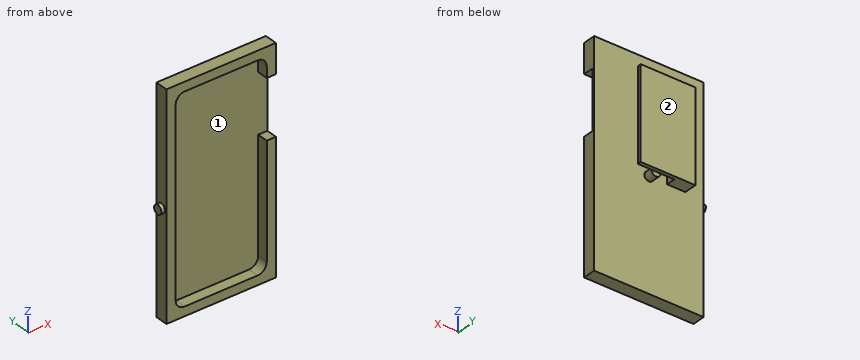
from build123d import *

# Parameters (mm, degrees)
F0_W      = 76.2
F0_H      = 152.4
F1_DEPTH  = 8.89
F3_DEPTH  = 7.62
F4_W      = 6.35
F4_H      = 40.64
F5_DEPTH  = 7.62
F7_DEPTH  = 2.54
F7_FACE_R = 3.175
F8_DEPTH  = 5.08
F9_R      = 3.175
F10_DEPTH = 6.35
F11_W     = 12.7
F11_H     = 63.5
F12_DEPTH = 8.89
F13_W     = 2.54
F13_H     = 63.5
F14_DEPTH = 25.4


with BuildPart() as f1:
    # F0 (on Front) → F1 (new body)
    with BuildSketch(Plane.XZ):
        with Locations((-38.1, 82.721622)):
            Rectangle(F0_W, F0_H)
    extrude(amount=F1_DEPTH)

    # F2 (on face) → F3 (cut)
    with BuildSketch(Plane.XZ.offset(8.89)):
        with BuildLine():
            ThreePointArc((-69.85, 19.221622), (-67.990128, 14.731494), (-63.5, 12.871622))
            Line((-63.5, 12.871622), (-12.7, 12.871622))
            ThreePointArc((-12.7, 12.871622), (-8.209872, 14.731494), (-6.35, 19.221622))
            Line((-6.35, 19.221622), (-6.35, 146.221622))
            ThreePointArc((-6.35, 146.221622), (-8.209872, 150.71175), (-12.7, 152.571622))
            Line((-12.7, 152.571622), (-50.255585, 152.571622))
            Line((-50.255585, 152.571622), (-63.5, 152.571622))
            ThreePointArc((-63.5, 152.571622), (-67.990128, 150.71175), (-69.85, 146.221622))
            Line((-69.85, 146.221622), (-69.85, 115.075722))
            Line((-69.85, 115.075722), (-69.85, 19.221622))
        make_face()
    extrude(amount=-F3_DEPTH, mode=Mode.SUBTRACT)

    # F4 (on face) → F5 (cut)
    with BuildSketch(Plane.XZ.offset(8.89)):
        with Locations((-3.175, 118.281622)):
            Rectangle(F4_W, F4_H)
    extrude(amount=-F5_DEPTH, mode=Mode.SUBTRACT)

    # F6 (on face) → F7 (cut)
    with BuildSketch(Plane(origin=(-76.2, 0, 0), x_dir=(0, -1, 0), z_dir=(-1, 0, 0))):
        with BuildLine():
            ThreePointArc((4.445, 76.371622), (6.64402, 77.326013), (7.548988, 79.545828))
            ThreePointArc((7.548988, 79.545828), (2.103956, 81.765643), (4.445, 76.371622))
        make_face()
    extrude(amount=-F7_DEPTH, mode=Mode.SUBTRACT)

    # F7_face (on face) → F8 (join)
    with BuildSketch(Plane(origin=(-73.66, -4.373988, 79.545828), x_dir=(0, -1, 0), z_dir=(-1, 0, 0))):
        Circle(F7_FACE_R)
    extrude(amount=F8_DEPTH)

    # F9 (on face) → F10 (join)
    with BuildSketch(Plane(origin=(0, 0, 0), x_dir=(-1, 0, 0), z_dir=(0, 1, 0))):
        with Locations((38.1, 82.721622)):
            Circle(F9_R)
    extrude(amount=F10_DEPTH)

    # F11 (on face) → F12 (join)
    with BuildSketch(Plane(origin=(0, 0, 0), x_dir=(-1, 0, 0), z_dir=(0, 1, 0))):
        with Locations((57.15, 114.471622)):
            Rectangle(F11_W, F11_H)
    extrude(amount=F12_DEPTH)

    # F13 (on face) → F14 (join)
    with BuildSketch(Plane.YZ.offset(-50.8)):
        with Locations((7.62, 114.471622)):
            Rectangle(F13_W, F13_H)
    extrude(amount=F14_DEPTH)


solid = f1.part
Here's how the part is built. I have some questions about the finished solid (model axes, mm). Face numbers are marked on the shaded views. Give positions to 0.01 mm unless a question says otherwise; leave off trailing zeros. Loops run counter-clockwise (first coordinate to the right, second up) from the corner with the lowest first, then second, coordinate; pieces in that order, holes last. Notation, with made-up numbers: (32.5, 73) -> (83.5, 73) arc R20 ccw to (83.5, 91) -> close; hole circle Ø5 at (-29.5, 8). An arc over 180 degrees is marked (long way). One line per item, written item: value.
Q1. Suppose I cut it at C-C on x = -38.1. Please give me the cut outline in (y, z), then the cut area to 3 significant figures.
Answers follow:
outline: (-8.89, 6.52) -> (0, 6.52) -> (0, 79.55) -> (6.35, 79.55) -> (6.35, 82.72) -> (8.89, 82.72) -> (8.89, 146.22) -> (6.35, 146.22) -> (6.35, 85.9) -> (0, 85.9) -> (0, 158.92) -> (-8.89, 158.92) -> (-8.89, 152.57) -> (-1.27, 152.57) -> (-1.27, 12.87) -> (-8.89, 12.87) -> close
area: 492 mm^2
Q2. Suppose I cut it at B-B on z = 68. Please give me the cut outline in (x, y), then the cut area to 3 significant figures.
Answers follow:
outline: (-76.2, -8.89) -> (-69.85, -8.89) -> (-69.85, -1.27) -> (-6.35, -1.27) -> (-6.35, -8.89) -> (0, -8.89) -> (0, 0) -> (-76.2, 0) -> close
area: 194 mm^2
Q3. Suppose I cut it at A-A on y = 4.5. Please give me the cut outline in (x, z) (3 decimals), then the cut area to 3 significant figures.
Answers follow:
outline: (-63.5, 82.722) -> (-50.8, 82.722) -> (-50.8, 146.222) -> (-63.5, 146.222) -> close; circle Ø6.35 at (-38.1, 82.722)
area: 838 mm^2
Q4. We'd pull the mould along X, two halves only. Please class the marked faces 1 and 2: pulls with the +X half, pulls with the -X half, needs draft (parallel to the pull), parting line crosses it, or undercut.
Answers follow:
face 1: undercut
face 2: needs draft
Q5. If I drill on line 1 along Y through (x, z) = (-39, 99); line 2 along Z through (x, y) = (-24, -3); line 3 along X through (y, z) = (-5.75, 52), over which ranges is the centre line in solid material (lowest first)?
Answers follow:
line 1: -1.27 to 0, 6.35 to 8.89
line 2: 6.52 to 12.87, 152.57 to 158.92
line 3: -76.2 to -69.85, -6.35 to 0
Q6. I'm going to push flat-ended pins straight in: pin 1 Ø3 at (y, z) = (-1, 60) entering from -X; pin 2 Ø4 at (y, z) = (6.5, 126.5) entering from -X; pin 3 Ø10 at (x, y) = (-36, 5.5) entering from -Z. Where does each tip first touch, or does it pass through?
Answers follow:
pin 1: x = -76.2
pin 2: x = -63.5
pin 3: z = 79.55
Q7. Suppose I cut it at D-D on y = -6. Please give me the cut outline in (x, z), then the cut area to 3 significant figures.
Answers follow:
outline: (-78.74, 76.82) -> (-76.2, 76.82) -> (-76.2, 6.52) -> (0, 6.52) -> (0, 97.96) -> (-6.35, 97.96) -> (-6.35, 19.22) arc R6.35 cw to (-12.7, 12.87) -> (-63.5, 12.87) arc R6.35 cw to (-69.85, 19.22) -> (-69.85, 146.22) arc R6.35 cw to (-63.5, 152.57) -> (-12.7, 152.57) arc R6.35 cw to (-6.35, 146.22) -> (-6.35, 138.6) -> (0, 138.6) -> (0, 158.92) -> (-76.2, 158.92) -> (-76.2, 82.27) -> (-78.74, 82.27) -> close
area: 2,530 mm^2
